Autodesk Inventor part; units mm, degrees
ref_plane "YZ Plane" through (0, 0, 0) normal (1, 0, 0) x (0, 1, 0)
ref_plane "XZ Plane" through (0, 0, 0) normal (0, 1, 0) x (-1, 0, 0)
ref_plane "XY Plane" through (0, 0, 0) normal (0, 0, 1) x (1, 0, 0)
sketch "Szkic1" plane through (0, 0, 0) normal (0, 1, 0) x (-1, 0, 0)
  line L0 (52.5, 25) -> (-52.5, 25)
  line L1 (-52.5, 25) -> (-52.5, -25)
  line L2 (-52.5, -25) -> (52.5, -25)
  line L3 (52.5, -25) -> (52.5, 25)
  line L4 (52.5, 25) -> (-52.5, -25) construction
  line L5 (-52.5, 25) -> (52.5, -25) construction
  point P0 (0, 0)
  dimension "d0" = 105
  dimension "d1" = 50
extrude "Wyciągnięcie proste1" add sketch "Szkic1" along normal blind 1.6
sketch "Szkic5" plane through (0, 1.6, 0) normal (0, 1, 0) x (1, 0, 0)
  circle A0 centre (-40.05, 11.85) radius 1.6
  circle A1 centre (-40.05, -11.85) radius 1.6
  circle A2 centre (40.05, 11.85) radius 1.6
  circle A3 centre (40.05, -11.85) radius 1.6
  point P0 (0, 0)
extrude "Wyciągnięcie proste4" cut sketch "Szkic5" against normal blind 10
sketch "Szkic6" plane through (0, 1.6, 0) normal (0, 1, 0) x (1, 0, 0)
  line L0 (52.5, 25) -> (-52.5, 25)
  line L1 (52.5, 25) -> (-52.5, 25)
  line L2 (-52.5, 25) -> (-52.5, 35)
  line L3 (-52.5, 35) -> (52.5, 35)
  line L4 (52.5, 35) -> (52.5, 25)
  point P0 (0, 0)
  point P1 (-52.5, 25)
  dimension "d15" = 10
extrude "Wyciągnięcie proste5" add sketch "Szkic6" against normal up to surface (1.6 mm away)
sketch "Szkic7" plane through (0, 1.6, 0) normal (0, 1, 0) x (1, 0, 0)
  arc A0 (35.2, -11.85) -> (44.9, -11.85) centre (40.05, -11.85) ccw
  arc A1 (46.9, -9) -> (44.9, -11) centre (46.9, -11) ccw
  line L0 (44.9, -11) -> (44.9, -11.85)
  line L1 (52.5, -9) -> (35.2, -9)
  line L2 (52.5, 9) -> (35.2, 9)
  arc A2 (44.9, 11) -> (46.9, 9) centre (46.9, 11) ccw
  arc A3 (44.9, 11.85) -> (35.2, 11.85) centre (40.05, 11.85) ccw
  line L3 (-52.5, -9) -> (-35.2, -9)
  arc A4 (-44.9, -11) -> (-46.9, -9) centre (-46.9, -11) ccw
  arc A5 (-44.9, -11.85) -> (-35.2, -11.85) centre (-40.05, -11.85) ccw
  line L4 (-52.5, 9) -> (-35.2, 9)
  arc A6 (-46.9, 9) -> (-44.9, 11) centre (-46.9, 11) ccw
  arc A7 (-35.2, 11.85) -> (-44.9, 11.85) centre (-40.05, 11.85) ccw
  line L5 (40.05, -16.7) -> (-40.05, -16.7)
  line L6 (52.5, 35) -> (-52.5, 35)
  circle A8 centre (11, -83.1715) radius 1.55
  circle A9 centre (-11, -83.1715) radius 1.55
  circle A10 centre (-11, -21.7) radius 1.55
  circle A11 centre (11, -21.7) radius 1.55
  circle A12 centre (-11, -21.7) radius 5
  circle A13 centre (11, -21.7) radius 5
  line L7 (16, -21.7) -> (16, -16.7)
  line L8 (-16, -21.7) -> (-16, -16.7)
  line L9 (11, -26.7) -> (-11, -26.7)
  circle A14 centre (40.05, 11.85) radius 1.6
  circle A15 centre (-40.05, 11.85) radius 1.6
  circle A16 centre (40.05, -11.85) radius 1.6
  circle A17 centre (-40.05, -11.85) radius 1.6
  line L10 (52.5, -25) -> (52.5, 35)
  line L11 (52.5, 35) -> (-52.5, 35)
  line L12 (-52.5, 35) -> (-52.5, -25)
  line L13 (-52.5, -25) -> (52.5, -25)
  arc A18 (-44.9, -11.85) -> (-35.2, -11.85) centre (-40.05, -11.85) ccw
  arc A19 (-44.9, -11.85) -> (-35.2, -11.85) centre (-40.05, -11.85) ccw
  line L14 (-44.9, -11.85) -> (-44.9, -11)
  point P0 (0, 0)
  point P1 (14.7563, -25)
  point P2 (-14.7563, -25)
  dimension "d18" = 3.1
  dimension "d19" = 3.1
  dimension "d20" = 10
  dimension "d21" = 10
extrude "Wyciągnięcie proste6" cut sketch "Szkic7" against normal blind 10 contours A0 L0 A1 L1 L10 L13 A13 L7 L5 | L8 A12 L13 L12 L3 A4 L14 A5 L5 | A10 | A11
sketch "Szkic8" plane through (0, 1.6, 0) normal (0, 1, 0) x (1, 0, 0)
  circle A0 centre (11, -21.7) radius 1.55
  circle A1 centre (-11, -21.7) radius 1.55
  arc A2 (14.7563, -25) -> (16, -21.7) centre (11, -21.7) ccw
  circle A3 centre (11, -21.7) radius 5
  line L0 (-14.7563, -25) -> (14.7563, -25)
  circle A4 centre (-11, -21.7) radius 5
  line L1 (11, -26.7) -> (-11, -26.7)
  point P0 (0, 0)
extrude "Wyciągnięcie proste7" add sketch "Szkic8" against normal up to surface (1.6 mm away) contours A3 L0 | L1 A4 L0 A3 | A4 L0 picked at (-10.008, -25.2393)
sketch "Szkic9" plane through (0, 1.6, 0) normal (0, 1, 0) x (1, 0, 0)
  circle A0 centre (11, 10.1285) radius 1.5
  circle A1 centre (-11, 10.1285) radius 1.5
  circle A2 centre (-15, 31) radius 1.6
  circle A3 centre (15, 31) radius 1.6
  line L0 (15, 31) -> (-15, 31)
  line L1 (52.5, 35) -> (-52.5, 35)
  point P0 (0, 0)
  point P1 (0, 35)
  point P2 (0, 31)
  dimension "d26" = 3.2
  dimension "d27" = 3.2
  dimension "d28" = 30
  dimension "d29" = 4
extrude "Wyciągnięcie proste8" cut sketch "Szkic9" against normal through all contours A2 | A3
sketch "Szkic10" plane through (0, 1.6, 0) normal (0, 1, 0) x (1, 0, 0)
  line L0 (-27.4, 5.9859) -> (-27.4, -5.9859)
  line L1 (-25.6, 5.9859) -> (-27.4, 5.9859)
  line L2 (-25.6, -5.9859) -> (-25.6, 5.9859)
  line L3 (-27.4, -5.9859) -> (-25.6, -5.9859)
  line L4 (27.4, -5.9859) -> (27.4, 5.9859)
  line L5 (25.6, -5.9859) -> (27.4, -5.9859)
  line L6 (25.6, 5.9859) -> (25.6, -5.9859)
  line L7 (27.4, 5.9859) -> (25.6, 5.9859)
  line L8 (-27.9, -6.4859) -> (-27.9, 6.4859)
  line L9 (-27.9, 6.4859) -> (-25.1, 6.4859)
  line L10 (-25.1, 6.4859) -> (-25.1, -6.4859)
  line L11 (-25.1, -6.4859) -> (-27.9, -6.4859)
  line L12 (25.1, -6.4859) -> (27.9, -6.4859)
  line L13 (27.9, -6.4859) -> (27.9, 6.4859)
  line L14 (27.9, 6.4859) -> (25.1, 6.4859)
  line L15 (25.1, 6.4859) -> (25.1, -6.4859)
  point P0 (0, 0)
  dimension "d32" = 0.5
  dimension "d33" = 0.5
extrude "Wyciągnięcie proste9" cut sketch "Szkic10" against normal blind 10 contours L1 L2 L3 L0 | L5 L6 L7 L4 | L8 L9 L10 L11 | L15 L14 L13 L12
sketch "Szkic11" plane through (0, 1.6, 0) normal (0, 1, 0) x (1, 0, 0)
  circle A0 centre (40.05, 11.85) radius 1.6
  line L0 (52.5, 9) -> (46.9, 9)
  line L1 (52.5, 9) -> (52.5, 6)
  line L2 (52.5, 6) -> (35.2, 6)
  line L3 (35.2, 11.85) -> (35.2, 6)
  arc A1 (44.9, 11.85) -> (35.2, 11.85) centre (40.05, 11.85) ccw
  line L4 (44.9, 11.85) -> (44.9, 11)
  arc A2 (44.9, 11) -> (46.9, 9) centre (46.9, 11) ccw
  circle A3 centre (-40.05, 11.85) radius 1.6
  line L5 (-35.2, 6) -> (-35.2, 11.85)
  line L6 (-52.5, 6) -> (-35.2, 6)
  line L7 (-52.5, 9) -> (-52.5, 6)
  line L8 (-52.5, 9) -> (-46.9, 9)
  arc A4 (-46.9, 9) -> (-44.9, 11) centre (-46.9, 11) ccw
  line L9 (-44.9, 11.85) -> (-44.9, 11)
  arc A5 (-35.2, 11.85) -> (-44.9, 11.85) centre (-40.05, 11.85) ccw
  line L10 (44.4767, 13.8317) -> (35, 35)
  line L11 (-52.5, 35) -> (52.5, 35)
  circle A6 centre (15, 31) radius 1.6
  line L12 (-45.0282, 12.5998) -> (-35, 35)
  circle A7 centre (-15, 31) radius 1.6
  line L13 (-27.9, 6.4859) -> (-25.1, 6.4859)
  line L14 (-25.1, 6.4859) -> (-25.1, -6.4859)
  line L15 (-25.1, -6.4859) -> (-27.9, -6.4859)
  line L16 (-27.9, -6.4859) -> (-27.9, 6.4859)
  line L17 (25.1, 6.4859) -> (27.9, 6.4859)
  line L18 (27.9, 6.4859) -> (27.9, -6.4859)
  line L19 (27.9, -6.4859) -> (25.1, -6.4859)
  line L20 (25.1, -6.4859) -> (25.1, 6.4859)
  circle A8 centre (15, 31) radius 1.6
  circle A9 centre (-15, 31) radius 1.6
  line L21 (46.9, -9) -> (52.5, -9)
  line L22 (52.5, -9) -> (52.5, 35)
  line L23 (52.5, 35) -> (-52.5, 35)
  line L24 (-52.5, 35) -> (-52.5, -9)
  line L25 (-52.5, -9) -> (-46.9, -9)
  arc A10 (-44.9, -11) -> (-46.9, -9) centre (-46.9, -11) ccw
  line L26 (-44.9, -11) -> (-44.9, -11.85)
  arc A11 (-44.9, -11.85) -> (-40.05, -16.7) centre (-40.05, -11.85) ccw
  line L27 (-40.05, -16.7) -> (-16, -16.7)
  line L28 (-16, -16.7) -> (-16, -21.7)
  arc A12 (-16, -21.7) -> (-11, -26.7) centre (-11, -21.7) ccw
  line L29 (-11, -26.7) -> (11, -26.7)
  arc A13 (11, -26.7) -> (16, -21.7) centre (11, -21.7) ccw
  line L30 (16, -21.7) -> (16, -16.7)
  line L31 (16, -16.7) -> (40.05, -16.7)
  arc A14 (40.05, -16.7) -> (44.9, -11.85) centre (40.05, -11.85) ccw
  line L32 (44.9, -11.85) -> (44.9, -11)
  arc A15 (46.9, -9) -> (44.9, -11) centre (46.9, -11) ccw
  circle A16 centre (11, -21.7) radius 1.55
  circle A17 centre (-11, -21.7) radius 1.55
  circle A18 centre (40.05, 11.85) radius 1.6
  circle A19 centre (-40.05, 11.85) radius 1.6
  circle A20 centre (40.05, -11.85) radius 1.6
  circle A21 centre (-40.05, -11.85) radius 1.6
  point P0 (0, 0)
  point P1 (-44.4767, 13.8317)
  point P2 (52.5, 35)
  dimension "d36" = 20
  dimension "d37" = 20
extrude "Wyciągnięcie proste10" cut sketch "Szkic11" against normal blind 10 contours L0 A2 L4 A1 L10 L11 L22 | L12 A5 L9 A4 L8 L24 L11
sketch "Szkic13" plane through (0, 1.6, 0) normal (0, 1, 0) x (1, 0, 0)
  arc A0 (-44.9, -11.85) -> (-40.05, -16.7) centre (-40.05, -11.85) ccw
  arc A1 (-16, -21.7) -> (-11, -26.7) centre (-11, -21.7) ccw
  arc A2 (11, -26.7) -> (16, -21.7) centre (11, -21.7) ccw
  arc A3 (40.05, -16.7) -> (44.9, -11.85) centre (40.05, -11.85) ccw
  line L0 (-50.1769, -13.4907) -> (-7.453, -28.2105)
  line L1 (7.6845, -28.1307) -> (52.6221, -12.6483)
  line L2 (-40.05, -16.7) -> (-16, -16.7)
  line L3 (-16, -16.7) -> (-16, -21.7)
  line L4 (16, -21.7) -> (16, -16.7)
  line L5 (16, -16.7) -> (40.05, -16.7)
  point P0 (0, 0)
  point P1 (12.6287, -26.4273)
  point P2 (41.6298, -16.4355)
  point P3 (-41.6298, -16.4355)
  point P4 (-12.6287, -26.4273)
extrude "Wyciągnięcie proste11" add sketch "Szkic13" against normal up to surface (1.6 mm away)
sketch "Szkic14" plane through (0, 1.6, 0) normal (0, 1, 0) x (1, 0, 0)
  circle A0 centre (-40.05, -11.85) radius 1.6
  circle A1 centre (40.05, -11.85) radius 1.6
  circle A2 centre (-40.05, 11.85) radius 1.6
  circle A3 centre (40.05, 11.85) radius 1.6
  circle A4 centre (-11, -21.7) radius 1.55
  circle A5 centre (11, -21.7) radius 1.55
  circle A6 centre (-15, 31) radius 1.6
  circle A7 centre (15, 31) radius 1.6
  line L0 (25.1, 6.4859) -> (27.9, 6.4859)
  line L1 (27.9, 6.4859) -> (27.9, -6.4859)
  line L2 (27.9, -6.4859) -> (25.1, -6.4859)
  line L3 (25.1, -6.4859) -> (25.1, 6.4859)
  line L4 (-27.9, 6.4859) -> (-25.1, 6.4859)
  line L5 (-25.1, 6.4859) -> (-25.1, -6.4859)
  line L6 (-25.1, -6.4859) -> (-27.9, -6.4859)
  line L7 (-27.9, -6.4859) -> (-27.9, 6.4859)
  line L8 (-35, 35) -> (-44.4767, 13.8317)
  arc A8 (-44.4767, 13.8317) -> (-44.9, 11.85) centre (-40.05, 11.85) ccw
  line L9 (-44.9, 11.85) -> (-44.9, 11)
  arc A9 (-46.9, 9) -> (-44.9, 11) centre (-46.9, 11) ccw
  line L10 (-46.9, 9) -> (-52.5, 9)
  line L11 (-52.5, 9) -> (-52.5, -9)
  line L12 (-52.5, -9) -> (-46.9, -9)
  arc A10 (-44.9, -11) -> (-46.9, -9) centre (-46.9, -11) ccw
  line L13 (-44.9, -11) -> (-44.9, -11.85)
  arc A11 (-44.9, -11.85) -> (-41.6298, -16.4355) centre (-40.05, -11.85) ccw
  line L14 (-41.6298, -16.4355) -> (-12.6287, -26.4273)
  arc A12 (-12.6287, -26.4273) -> (-11, -26.7) centre (-11, -21.7) ccw
  line L15 (-11, -26.7) -> (11, -26.7)
  arc A13 (11, -26.7) -> (12.6287, -26.4273) centre (11, -21.7) ccw
  line L16 (12.6287, -26.4273) -> (41.6298, -16.4355)
  arc A14 (41.6298, -16.4355) -> (44.9, -11.85) centre (40.05, -11.85) ccw
  line L17 (44.9, -11.85) -> (44.9, -11)
  arc A15 (46.9, -9) -> (44.9, -11) centre (46.9, -11) ccw
  line L18 (46.9, -9) -> (52.5, -9)
  line L19 (52.5, -9) -> (52.5, 9)
  line L20 (52.5, 9) -> (46.9, 9)
  arc A16 (44.9, 11) -> (46.9, 9) centre (46.9, 11) ccw
  line L21 (44.9, 11) -> (44.9, 11.85)
  arc A17 (44.9, 11.85) -> (44.4767, 13.8317) centre (40.05, 11.85) ccw
  line L22 (44.4767, 13.8317) -> (35, 35)
  line L23 (35, 35) -> (-35, 35)
  point P0 (0, 0)
properties part number "ty"
The model under review builds one solid part; all positions refer to its coordinate system, in mm. Coordinates: 2 decimals unless noted, no trailing zeros. Write each loop counter-clockwise with the first axis right and the second up, starting at its lowest first coordinate (ties: lowest second). Pieces come first, ordered by that corner, then holes. Notation, with made-up numbers: (22, 20) -> (76, 20) arc R26 cw to (76, 52) -> close; hole circle Ø6 at (76.25, -5.5). An arc over 180 degrees is marked (long way). Answer in a Markdown table with one row per item.
1. Wall thickness on probe 1 along X at (y, z) = (0.75, 11.85); probe 2 along X at (y, z) = (0.25, 4); probe 3 along Z at (x, y) = (11, 0.6): over which ranges is each line inside the solid? List them lowest first. Write a range as [from, to].
Answers below:
| item | result |
|---|---|
| probe 1 | x = [-44.9, -41.65], [-38.45, 38.45], [41.65, 44.9] |
| probe 2 | x = [-52.5, -27.9], [-25.1, 25.1], [27.9, 52.5] |
| probe 3 | z = [-35, 20.15], [23.25, 26.7] |
2. Draft analysis for pull direction Z (two halves, no side actions). For faces 1 (the cylindrical face through (41.576, 0.811, -12.331)), 2 (the cylindrical face through (-45.5, 0.81, -9.57)), 3 (the cylindrical face through (-45.47, 0.81, 9.6)), state which applies: +Z half, -Z half, draft (parallel to the pull), parting line (faces both ways), or undercut.
Answers below:
| item | result |
|---|---|
| face 1 | undercut |
| face 2 | -Z half |
| face 3 | +Z half |
3. We need section A-A, the plane z = -1.5. State the section outline as (x, y) points, and give its area (3 significant figures).
Answers below:
| item | result |
|---|---|
| outline | (-52.5, 0) -> (-27.9, 0) -> (-27.9, 1.6) -> (-52.5, 1.6) -> close; (-25.1, 0) -> (25.1, 0) -> (25.1, 1.6) -> (-25.1, 1.6) -> close; (27.9, 0) -> (52.5, 0) -> (52.5, 1.6) -> (27.9, 1.6) -> close |
| area | 159 mm^2 |
4. We need section B-B, the plane x = 40.05. State the section outline as (y, z) points, and give its area (3 significant figures).
Answers below:
| item | result |
|---|---|
| outline | (0, -23.72) -> (1.6, -23.72) -> (1.6, -13.45) -> (0, -13.45) -> close; (0, -10.25) -> (1.6, -10.25) -> (1.6, 10.25) -> (0, 10.25) -> close; (0, 13.45) -> (1.6, 13.45) -> (1.6, 16.98) -> (0, 16.98) -> close |
| area | 54.9 mm^2 |
5. We need section C-C, the plane y = 1.1. Give the number of separate pieces and of enclosed holes in the cut face, and give its area (3 significant figures).
Answers below:
| item | result |
|---|---|
| separate pieces | 1 |
| enclosed holes | 10 |
| area | 5,080 mm^2 |
6. Clearance check with flat-ended pins moving along their axes: pin 1 Ø1.9 at (x, z) = (15, -31) entering from +Y; pin 2 Ø1 at (x, z) = (15.5, 10.5) entering from -Y; pin 3 Ø0.9 at (y, z) = (0.5, 11.5) entering from +X; pin 4 Ø0.7 at (y, z) = (1, 11.5) entering from -X. State where each tip first meets the part, or that it passes through.
Answers below:
| item | result |
|---|---|
| pin 1 | passes through |
| pin 2 | stops at y = 0 |
| pin 3 | stops at x = 44.9 |
| pin 4 | stops at x = -44.9 |
